Answer from the drawing. Dimensions are ordinates in mm from the lowest x, y and z of the part. A direction names the side the tool comes from. Round coordinates to 2 decimals unless told otherwise and drop trailing zeros. Loops run counter-clockwise (first coordinate to the right, second up) from the corner with the lowest first, then second, coordinate; pieces in that order, holes last. Notation, with made-up numbers: (29.25, -2.75) - (81.25, -2.75) arc R34 cw to (81.25, 28.25) - close; hole circle Ø5 at (22, 52.5). An arc over 180 degrees is marked (long way). Return JSON: item names as keys, results as strings.
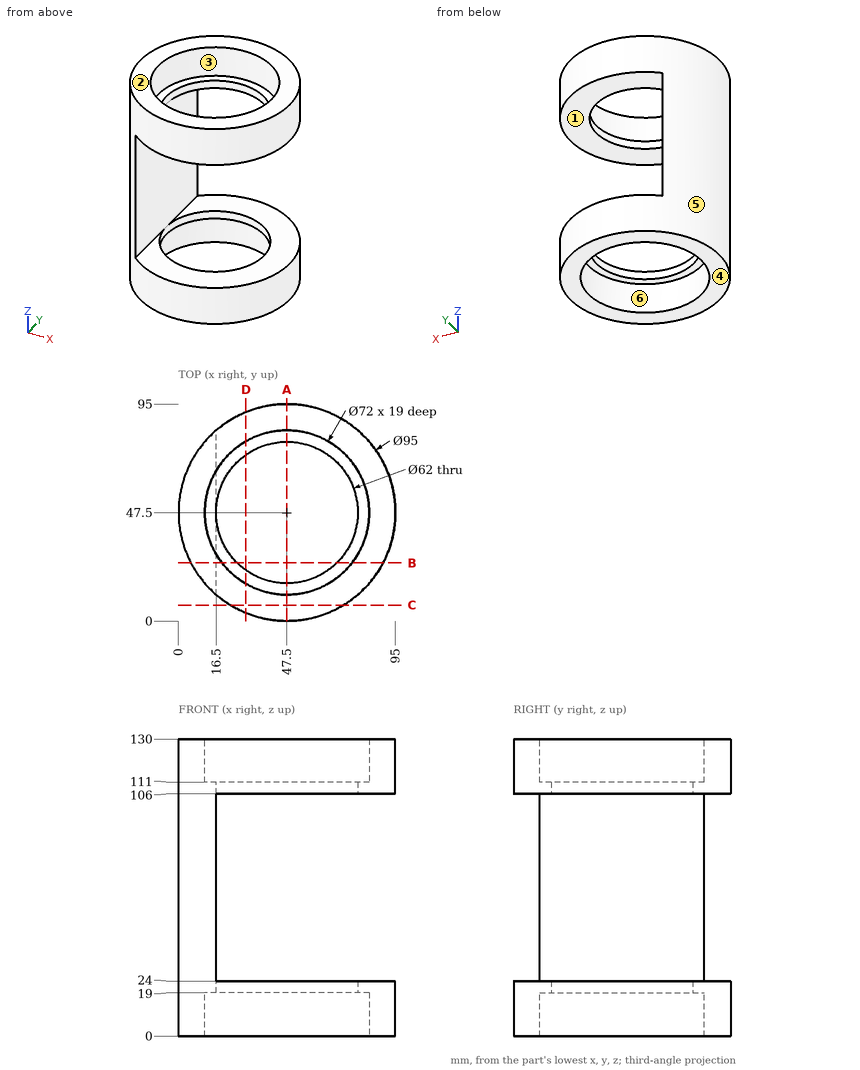
1) Section A-A (x = 47.5) is taken. Give the vertices of the cut face in (y, z).
Verdict:
{"outline": "(0, 0) - (11.5, 0) - (11.5, 19) - (16.5, 19) - (16.5, 24) - (0, 24) - close; (0, 106) - (16.5, 106) - (16.5, 111) - (11.5, 111) - (11.5, 130) - (0, 130) - close; (78.5, 19) - (83.5, 19) - (83.5, 0) - (95, 0) - (95, 24) - (78.5, 24) - close; (78.5, 106) - (95, 106) - (95, 130) - (83.5, 130) - (83.5, 111) - (78.5, 111) - close"}
2) Flat-ended cylindrical pins translate along their axes: pin 1 (21.5 mm diameter, centred on x = 61, y = 44, fed in from -Z); pin 2 (12 mm diameter, centred on x = 25.5, y = 31.5, fed in from +Z); pin 3 (6 mm diameter, centred on y = 37, z = 33, fed in from -X); pin 4 (3 mm diameter, centred on y = 55, z = 100.5, fed in from +X). Find the tip coordinate at first contact, or state that the pin passes through.
Verdict:
{"pin 1": "passes through", "pin 2": "stops at z = 111", "pin 3": "stops at x = 0.6", "pin 4": "stops at x = 16.5"}
3) Section C-C (y = 7) is taken. Give the vertices of the cut face in (x, z).
Verdict:
{"outline": "(22.68, 0) - (72.32, 0) - (72.32, 24) - (22.68, 24) - close; (22.68, 106) - (72.32, 106) - (72.32, 130) - (22.68, 130) - close"}
4) Determine the mould class of the marked faces 3, 4, 5 and 6 for opening direction Y: pulls with the +Y half, pulls with the -Y half, needs draft (parallel to the pull), parting line crosses it, or undercut.
Verdict:
{"face 3": "undercut", "face 4": "needs draft", "face 5": "parting line crosses it", "face 6": "undercut"}
5) A tool of negligible diameter and unlimited length cuts with its end or side. For the marked faces 1 and 2, from which of +Z, -Z, +X, -X, +Y, -Y can it reach the whole face along a straight path? Write none if from no direction.
Verdict:
{"face 1": "+X, +Y, -Y", "face 2": "+Z, +X, -X, +Y, -Y"}
6) Section B-B (y = 25.5) is taken. Give the vertices of the cut face in (x, z).
Verdict:
{"outline": "(5.4, 0) - (19, 0) - (19, 19) - (25.66, 19) - (25.66, 24) - (16.5, 24) - (16.5, 106) - (25.66, 106) - (25.66, 111) - (19, 111) - (19, 130) - (5.4, 130) - close; (69.34, 19) - (76, 19) - (76, 0) - (89.6, 0) - (89.6, 24) - (69.34, 24) - close; (69.34, 106) - (89.6, 106) - (89.6, 130) - (76, 130) - (76, 111) - (69.34, 111) - close"}
7) Find the intervals of material crossed by L1, parallel to Y at x = 47, z = 21; L2, parallel to Z at x = 75.5, y = 67; L3, parallel to Z at x = 84.5, y = 38, in increasing order.
Verdict:
{"L1": "y = 0 to 16.5, 78.5 to 95", "L2": "z = 19 to 24, 106 to 111", "L3": "z = 0 to 24, 106 to 130"}
8) Section D-D (x = 29.5) is taken. Give the vertices of the cut face in (y, z), and give its area (3 significant figures).
Verdict:
{"outline": "(3.54, 0) - (16.32, 0) - (16.32, 19) - (22.26, 19) - (22.26, 24) - (3.54, 24) - close; (3.54, 106) - (22.26, 106) - (22.26, 111) - (16.32, 111) - (16.32, 130) - (3.54, 130) - close; (72.74, 19) - (78.68, 19) - (78.68, 0) - (91.46, 0) - (91.46, 24) - (72.74, 24) - close; (72.74, 106) - (91.46, 106) - (91.46, 130) - (78.68, 130) - (78.68, 111) - (72.74, 111) - close", "area": "1,350 mm2"}
